Geometry check sheet. Reference: the model listing, model coordinates, mm. Face numbers are marked on the shaded views. A direction names the side the tool comes from. Round coordinates to 2 decimals unless told otherwise and drop trailing zeros. Write each loop counter-clockwise with the first axis right and the second up, starting at its lowest first coordinate (ties: lowest second). Pieces come first, ordered by that corner, then holes. Notation, with made-up numbers: M 76.25,12 L 111.25,12 A23 cw 111.25,47 Z; hole C 20.25,61 d9. An arc over 180 degrees is marked long. Answer in a Markdown table with one row per item. Add a question column.
Autodesk Inventor part; units mm, degrees
ref_plane "YZ Plane" through (0, 0, 0) normal (1, 0, 0) x (0, 1, 0)
ref_plane "XZ Plane" through (0, 0, 0) normal (0, 1, 0) x (-1, 0, 0)
ref_plane "XY Plane" through (0, 0, 0) normal (0, 0, 1) x (1, 0, 0)
sketch "Sketch1" plane through (0, 0, 0) normal (0, 0, 1) x (1, 0, 0)
  circle A0 centre (0, 0) radius 17.75
  circle A1 centre (0, 0) radius 20
  dimension "d0" = 35.5
  dimension "d1" = 40
extrude "Extrusion1" add sketch "Sketch1" along normal blind 7
sketch "Sketch2" plane through (0, 0, 0) normal (0, 0, -1) x (-1, 0, 0)
  circle A0 centre (0, 0) radius 20
extrude "Extrusion2" add sketch "Sketch2" along normal blind 5
sketch "Sketch3" plane through (0, 0, -5) normal (0, 0, -1) x (-1, 0, 0)
  circle A0 centre (0, 0) radius 20
  line L0 (-17.5997, 9.5) -> (17.5997, 9.5)
  line L1 (-17.5997, -9.5) -> (17.5997, -9.5)
  circle A1 centre (0, 0) radius 20
  line L2 (58, 0) -> (-33, 0)
  dimension "d6" = 19
  dimension "d7" = 9.5
extrude "Extrusion3" cut sketch "Sketch3" against normal through all contours L0 A0 | A0 L1
sketch "Sketch4" plane through (0, 0, -5) normal (0, 0, -1) x (-1, 0, 0)
  arc A0 (17.5997, -9.5) -> (17.5997, 9.5) centre (0, 0) ccw
  line L0 (17.5997, 9.5) -> (45, 9.5)
  line L1 (45, 9.5) -> (45, -9.5)
  arc A1 (17.5997, -9.5) -> (17.5997, 9.5) centre (0, 0) ccw
  line L2 (45, -9.5) -> (17.5997, -9.5)
  line L3 (14.9937, -9.5) -> (-14.9937, -9.5)
  arc A2 (-14.9937, 9.5) -> (-14.9937, -9.5) centre (0, 0) ccw
  line L4 (-14.9937, 9.5) -> (14.9937, 9.5)
  arc A3 (14.9937, -9.5) -> (14.9937, 9.5) centre (0, 0) ccw
  dimension "d10" = 90
  dimension "d11" = 45
extrude "Extrusion4" add sketch "Sketch4" against normal blind 5 contours A0 L0 L1 L2
sketch "Sketch5" plane through (0, 0, 0) normal (0, 0, 1) x (1, 0, 0)
  line L0 (17.5997, -9.5) -> (-45, -9.5)
  line L1 (-45, 9.5) -> (17.5997, 9.5)
  line L2 (-45, -9.5) -> (-40, -9.5)
  line L3 (-40, -9.5) -> (-40, 9.5)
  line L4 (-40, 9.5) -> (-45, 9.5)
  line L5 (-45, 9.5) -> (-45, -9.5)
  point P0 (0, 0)
  dimension "d14" = 5
extrude "Extrusion5" add sketch "Sketch5" along normal blind 15
sketch "Sketch6" plane through (-40, -9.5, 0) normal (1, 0, 0) x (0, 0, -1)
  point P0 (0, 9.5)
sketch "Sketch7" plane through (-45, -9.5, -5) normal (-1, 0, 0) x (0, 0, 1)
  line L0 (12, 19) -> (12, 0)
  circle A0 centre (12, 9.5) radius 2.25
  point P0 (5, 9.5)
  dimension "d17" = 4.5
extrude "Extrusion6" cut sketch "Sketch7" against normal up to surface (5 mm away)
fillet "Fillet1" radius 2 1 edges at (-40, 0, 0)
fillet "Fillet2" radius 2 1 edges at (-40, 0, 15)
fillet "Fillet3" radius 2 2 edges at (-17.75, 0, 7) (17.75, 0, 7)
fillet_without_effect "Fillet4"
fillet "Fillet6" radius 2 1 edges at (-20, 0, 0)
properties part number "Lid_holder"
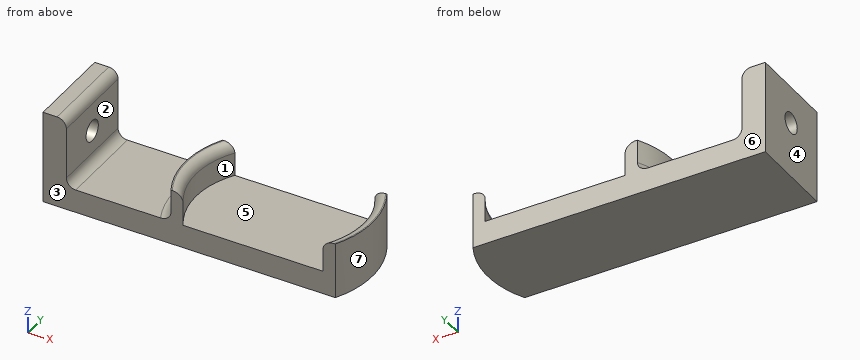
Item 1: Section check A-A, the plane y = 0. Record the boundary of the cut face in (x, z).
Item 2: Section check B-B, the plane z = 1.25. Record the boundary of the cut face in (x, y).
Item 3: Gauge pin test, flat ends, axial feed: pin 1 Ø5.5 at (y, z) = (3.5, 6) entering from +X; pin 2 Ø1.3 at (x, y) = (18, 2) entering from +Z; pin 3 Ø3 at (x, y) = (2, 6.5) entering from +Z; pin 4 Ø12 at (x, z) = (-22, 7.5) entering from +Y. Record the tip position at first contact, or that the pin passes through.
Item 4: Access from +Z, -Z, +X, -X, +Y, -Y to the whole of each face (thin tool, end or side, straight path). Record for the marked faces 1, 2 and 3.
Item 5: Section check C-C, the plane z = 6.25. Record the boundary of the cut face in (x, y), and give its area (3 significant figures).
Item 6: Section check D-D, the plane x = -25. Record the boundary of the cut face in (y, z).
Item 7: Mould release check, pull along X, two halves, no side actions. Record for the marked faces 4, 5, 6 and 7: +X half, -X half, draft (parallel to the pull), parting line (faces both ways), or undercut.
Item 8: Scan lines: probe 1 along Y at (x, z) = (-42.4, 7); probe 2 along X at (y, z) = (3.5, 4.5); probe 3 along X at (y, z) = (-5.25, 5.25). Record each from-to range of solid material in increasing order. Write a range as from..to.
Result sheet:
| question | item | result |
|---|---|---|
| 1 | outline | M -45,-5 L 20,-5 L 20,7 L 19.75,7 A2 ccw 17.75,5 L 17.75,0 L -17.75,0 L -17.75,5 A2 ccw -19.75,7 L -20,7 L -20,2 A2 cw -22,0 L -38,0 A2 cw -40,2 L -40,4.75 L -45,4.75 Z; M -45,9.25 L -40,9.25 L -40,13 A2 ccw -42,15 L -45,15 Z |
| 2 | outline | M -45,-9.5 L -39.85,-9.5 L -39.85,9.5 L -45,9.5 Z; M -17.77,-9.5 L -14.99,-9.5 A17.75 cw -14.99,9.5 L -17.77,9.5 A20.15 ccw Z; M 14.99,-9.5 L 17.6,-9.5 A20 ccw 17.6,9.5 L 14.99,9.5 A17.75 cw Z |
| 3 | pin 1 | stops at x = 19.99 |
| 3 | pin 2 | stops at z = 6.74 |
| 3 | pin 3 | stops at z = 0 |
| 3 | pin 4 | stops at y = 9.5 |
| 4 | face 1 | +Z |
| 4 | face 2 | +Z, +Y, -Y |
| 4 | face 3 | +Z, -Z, +X, -X, -Y |
| 5 | outline | M -45,-9.5 L -40,-9.5 L -40,-2.12 L -45,-2.12 Z; M -45,2.12 L -40,2.12 L -40,9.5 L -45,9.5 Z; M -17.6,-9.5 L -15.51,-9.5 A18.19 cw -15.51,9.5 L -17.6,9.5 A20 ccw Z; M 15.51,-9.5 L 17.6,-9.5 A20 ccw 17.6,9.5 L 15.51,9.5 A18.19 cw Z |
| 5 | area | 146 mm^2 |
| 6 | outline | M -9.5,-5 L 9.5,-5 L 9.5,0 L -9.5,0 Z |
| 7 | face 4 | -X half |
| 7 | face 5 | undercut |
| 7 | face 6 | draft |
| 7 | face 7 | +X half |
| 8 | probe 1 | y = -9.5..-2.25, 2.25..9.5 |
| 8 | probe 2 | x = -45..-40, -19.69..-17.4, 17.4..19.69 |
| 8 | probe 3 | x = -45..-40, -19.3..-16.97, 16.97..19.3 |
